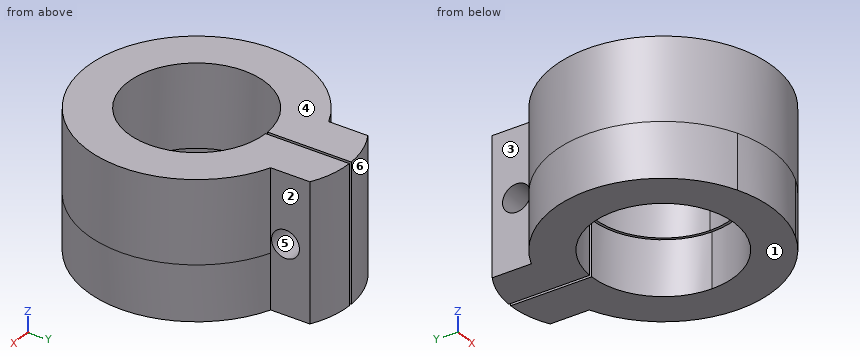
```python
from build123d import *

# Parameters (mm, degrees)
SKETCH_1_R          = 3.5
SKETCH_1_R_2        = 13
EXTRUDE_2_DEPTH     = 10
SKETCH_2_R          = 12.5
EXTRUDE_3_DEPTH     = 15
SKETCH_3_W          = 0.517195108
SKETCH_3_H          = 18.726193104
CUT_EXTRUDE_1_DEPTH = 26
SKETCH_4_R          = 2.5
CUT_EXTRUDE_2_DEPTH = 43.740275714
CUT_EXTRUDE_3_DEPTH = 10


with BuildPart() as part:
    # 草图1 → 凸台-拉伸2 (new body)
    with BuildSketch(Plane.XY):
        with BuildLine():
            Line((-35, -7), (-7.740275714, -18.44147857))
            ThreePointArc((-7.740275714, -18.44147857), (0, -20), (7.740275714, -18.44147857))
            Line((7.740275714, -18.44147857), (35, -7))
            Line((35, -7), (35, 7))
            Line((35, 7), (7.740275714, 18.44147857))
            Line((7.740275714, 18.44147857), (7.740275714, 25.44147857))
            ThreePointArc((7.740275714, 25.44147857), (0, 27.494244152), (-7.740275714, 25.44147857))
            Line((-7.740275714, 25.44147857), (-7.740275714, 18.44147857))
            Line((-7.740275714, 18.44147857), (-35, 7))
            Line((-35, 7), (-35, -7))
        make_face()
        with Locations((-28, 0)):
            Circle(SKETCH_1_R, mode=Mode.SUBTRACT)
        Circle(SKETCH_1_R_2, mode=Mode.SUBTRACT)
        with Locations((28, 0)):
            Circle(SKETCH_1_R, mode=Mode.SUBTRACT)
    extrude(amount=EXTRUDE_2_DEPTH)

    # 草图2 → 凸台-拉伸3 (add)
    with BuildSketch(Plane.XY.offset(10)):
        with BuildLine():
            Line((-7.740275714, 18.44147857), (-7.740275714, 25.44147857))
            ThreePointArc((-7.740275714, 25.44147857), (0, 27.494244152), (7.740275714, 25.44147857))
            Line((7.740275714, 25.44147857), (7.740275714, 18.44147857))
            ThreePointArc((7.740275714, 18.44147857), (0, -20), (-7.740275714, 18.44147857))
        make_face()
        Circle(SKETCH_2_R, mode=Mode.SUBTRACT)
    extrude(amount=EXTRUDE_3_DEPTH)

    # 草图3 → 切除-拉伸1 (cut, through all)
    with BuildSketch(Plane.XY.offset(25)):
        with Locations((0, 21.741202931)):
            Rectangle(SKETCH_3_W, SKETCH_3_H)
    extrude(amount=-CUT_EXTRUDE_1_DEPTH, mode=Mode.SUBTRACT)

    # 草图4 → 切除-拉伸2 (cut, through all)
    with BuildSketch(Plane(origin=(7.740275714, 0, 0), x_dir=(0, 0, -1), z_dir=(1, 0, 0))):
        with Locations((-12.5, 21.086423576)):
            Circle(SKETCH_4_R)
    extrude(amount=-CUT_EXTRUDE_2_DEPTH, mode=Mode.SUBTRACT)

    # 草图6 → 切除-拉伸3 (cut)
    with BuildSketch(Plane.XY.offset(10)):
        with BuildLine():
            Line((-7.740275714, 18.44147857), (-35, 7))
            Line((-35, 7), (-35, -7))
            Line((-35, -7), (-7.740275714, -18.44147857))
            ThreePointArc((-7.740275714, -18.44147857), (-20, 0), (-7.740275714, 18.44147857))
        make_face()
        with BuildLine():
            Line((7.740275714, -18.44147857), (35, -7))
            Line((35, -7), (35, 7))
            Line((35, 7), (7.740275714, 18.44147857))
            ThreePointArc((7.740275714, 18.44147857), (20, 0), (7.740275714, -18.44147857))
        make_face()
    extrude(amount=-CUT_EXTRUDE_3_DEPTH, mode=Mode.SUBTRACT)


solid = part.part
```
Verification items for the finished model (mm, model axes). Face numbers are marked on the shaded views. A direction names the side the tool comes from. Give positions to 0.01 mm unless a question says otherwise; leave off trailing zeros. Loops run counter-clockwise (first coordinate to the right, second up) from the corner with the lowest first, then second, coordinate; pieces in that order, holes last.
1. Go/stop test with flat-tipped pins: pin 1 Ø12 at (y, z) = (1.5, 9.5) entering from -X; pin 2 Ø8 at (y, z) = (21.09, 12.5) entering from +X; pin 3 Ø5.5 at (y, z) = (21, 16.5) entering from -X; pin 4 Ø22.5 at (x, y) = (0, 0) entering from -Z. Record where each tip stops, or that it passes through.
2. Set-up check for the marked faces 1, 2 and 3: record each of +Z, -Z, +X, -X, +Y, -Y from which the full face is reachable in a straight line by a thin tool's end or side.
3. Section check C-C, the plane z = 12.5. Enter the section's corners in (x, y).
4. Thickness scan on line 1 (Y direction, x = 1.5, z = 10.5); line 2 (X direction, y = 22, z = 9); line 3 (Y direction, x = -6, z = 12.5). Record the ranges inside material, lowest first.
5. Section check B-B, the plane z = 6.75. Enter the section's corners in (x, y).
6. Mould release check, pull along Y, two halves, no side actions. Record for the marked faces 4, 5 and 6: released by +Y, released by -Y, zero draft, split by the parting line, or undercut.
7. Section check D-D, the plane y = -10.5. Enter the section's corners in (x, z).
8. Section check A-A, the plane x = -3. Enter the section's corners in (y, z).
Geometry says:
1. pin 1: stops at x = -20
1. pin 2: stops at x = 10.39
1. pin 3: stops at x = -8.18
1. pin 4: passes through
2. face 1: -Z, +X, -X, +Y, -Y
2. face 2: +Z, -Z, +X, +Y
2. face 3: +Z, -Z, -X, +Y
3. outline: (-7.74, 18.44) arc R20 ccw (long way) to (7.74, 18.44) - (7.74, 18.59) - (0.26, 18.59) - (0.26, 12.5) arc R12.5 cw (long way) to (-0.26, 12.5) - (-0.26, 18.59) - (-7.74, 18.59) - close; (-7.74, 23.59) - (-0.26, 23.59) - (-0.26, 27.49) arc R15.62 ccw to (-7.74, 25.44) - close; (0.26, 23.59) - (7.74, 23.59) - (7.74, 25.44) arc R15.62 ccw to (0.26, 27.49) - close
4. line 1: y = -19.94 to -12.41, 12.41 to 19.59, 22.59 to 27.42
4. line 2: x = -7.74 to -0.26, 0.26 to 7.74
4. line 3: y = -19.08 to -10.97, 10.97 to 18.59, 23.59 to 26.3
5. outline: (-7.74, 18.44) arc R20 ccw (long way) to (7.74, 18.44) - (7.74, 25.44) arc R15.62 ccw to (0.26, 27.49) - (0.26, 13) arc R13 cw (long way) to (-0.26, 13) - (-0.26, 27.49) arc R15.62 ccw to (-7.74, 25.44) - close
6. face 4: zero draft
6. face 5: undercut
6. face 6: released by +Y
7. outline: (-17.02, 0) - (-7.66, 0) - (-7.66, 10) - (-6.78, 10) - (-6.78, 25) - (-17.02, 25) - close; (6.78, 10) - (7.66, 10) - (7.66, 0) - (17.02, 0) - (17.02, 25) - (6.78, 25) - close
8. outline: (-19.77, 0) - (-12.65, 0) - (-12.65, 10) - (-12.13, 10) - (-12.13, 25) - (-19.77, 25) - close; (12.13, 10) - (12.65, 10) - (12.65, 0) - (27.2, 0) - (27.2, 25) - (12.13, 25) - close; hole circle Ø5 at (21.09, 12.5)
